The listing builds one solid part. Answer for the finished solid, in the listing's coordinates (mm). Face numbers are marked on the shaded views. Give positions to 0.01 mm unless a question says otherwise; leave off trailing zeros. Loops run counter-clockwise (first coordinate to the right, second up) from the corner with the lowest first, then second, coordinate; pieces in that order, holes last. Notation, with made-up numbers: M 39,-25.5 L 88,-25.5 A8 cw 88,-13.5 Z; hole C 34,37 d4. An arc over 180 degrees is marked long. Use one line per item in the form item = value. Start each with the question number.
1. The part is cut by section B-B (z = 1.75). Write down the section's boundary in (x, y), and give its area (3 significant figures).
2. The mould has two halves that part along X. Classify the marked faces 1, 2, 3 and 4: released by +X, released by -X, zero draft, split by the parting line, or undercut.
3. The part is cut by section C-C (y = 5). Write down the section's boundary in (x, z).
4. The part is cut by section A-A (y = 15). Write down the section's boundary in (x, z).
5. Each of these flat-tipped pins is pushed along its axis until it touches: pin 1 Ø2 at (x, y) = (1.5, 15.5) entering from -Z; pin 2 Ø12 at (x, y) = (4, 26.5) entering from -Z; pin 3 Ø2.5 at (x, y) = (5, -5) entering from +Z; pin 4 Ø1.8 at (x, y) = (-5, -5) entering from -Z. Where does it stop, or does it pass through?
6. Straight lines are drawn through the part: line 1 (Y direction, x = 0, z = 3.85); line 2 (Y direction, x = 0, z = 1.7); line 3 (X direction, y = 5, z = 2.2). For each, find the intervals that lie inside material, in ascending order. Write a range as from..to.
7. The part is cut by section D-D (x = -0.5). Write down the section's boundary in (y, z).
from build123d import *

# Parameters (mm, degrees)
SKETCH2_R           = 10
SKETCH2_R_2         = 1
SKETCH2_R_3         = 1.5
BOSS_EXTRUDE1_DEPTH = 5
SKETCH5_R           = 2
SKETCH5_R_2         = 1
CUT_EXTRUDE2_DEPTH  = 2
SKETCH6_R           = 3.5
CUT_EXTRUDE3_DEPTH  = 3


with BuildPart() as part:
    # Sketch2 → Boss-Extrude1 (new body)
    # profile 1 of 2: a face of its own
    with BuildSketch(Plane.XY):
        Circle(SKETCH2_R)
        with Locations((5, -5)):
            Circle(SKETCH2_R_2, mode=Mode.SUBTRACT)
        with Locations((-5, -5)):
            Circle(SKETCH2_R_2, mode=Mode.SUBTRACT)
        with Locations((5, 5)):
            Circle(SKETCH2_R_2, mode=Mode.SUBTRACT)
        with Locations((-5, 5)):
            Circle(SKETCH2_R_2, mode=Mode.SUBTRACT)
    # profile 2 of 2: a face of its own
    with BuildSketch(Plane.XY):
        with BuildLine():
            Line((-10, 40), (-10, 0))
            ThreePointArc((-10, 0), (0, 10), (10, 0))
            Line((10, 0), (10, 40))
            Line((10, 40), (-10, 40))
        make_face()
        with Locations((0, 15)):
            Circle(SKETCH2_R_3, mode=Mode.SUBTRACT)
        with Locations((0, 35)):
            Circle(SKETCH2_R_3, mode=Mode.SUBTRACT)
    extrude(amount=BOSS_EXTRUDE1_DEPTH)

    # Sketch5 → Cut-Extrude2 (cut)
    with BuildSketch(Plane.XY.offset(5)):
        with Locations((-5, 5)):
            Circle(SKETCH5_R)
        with Locations((5, 5)):
            Circle(SKETCH5_R)
        with Locations((5, -5)):
            Circle(SKETCH5_R)
        with Locations((-5, -5)):
            Circle(SKETCH5_R)
        with Locations((0, 3)):
            Circle(SKETCH5_R_2)
        with Locations((-3, 0)):
            Circle(SKETCH5_R_2)
        with Locations((3, 0)):
            Circle(SKETCH5_R_2)
        with Locations((0, -3)):
            Circle(SKETCH5_R_2)
    extrude(amount=-CUT_EXTRUDE2_DEPTH, mode=Mode.SUBTRACT)

    # Sketch6 → Cut-Extrude3 (cut)
    with BuildSketch(Plane(origin=(0, 0, 0), x_dir=(-1, 0, 0), z_dir=(0, 0, -1))):
        with Locations((0, 35)):
            Circle(SKETCH6_R)
        with Locations((0, 15)):
            Circle(SKETCH6_R)
    extrude(amount=-CUT_EXTRUDE3_DEPTH, mode=Mode.SUBTRACT)


solid = part.part
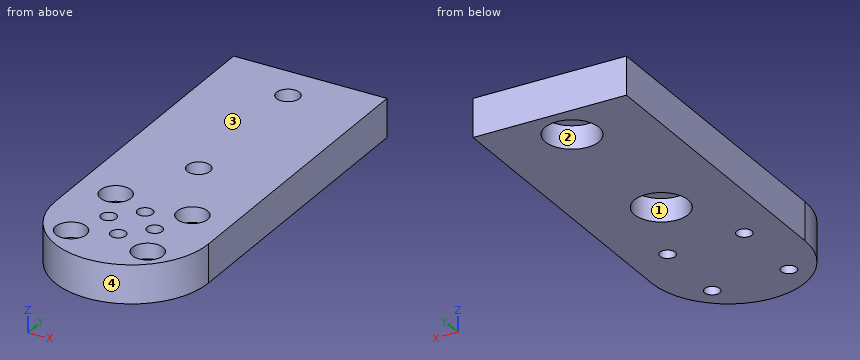
Derived:
q1.outline = M -10,0 A10 ccw 10,0 L 10,40 L -10,40 Z; hole C -5,-5 d2; hole C -5,5 d2; hole C 0,15 d7; hole C 0,35 d7; hole C 5,-5 d2; hole C 5,5 d2
q1.area = 868 mm2
q2.face_1 = undercut
q2.face_2 = undercut
q2.face_3 = zero draft
q2.face_4 = split by the parting line
q3.outline = M -10,0 L -6,0 L -6,3 L -7,3 L -7,5 L -10,5 Z; M -4,0 L 4,0 L 4,3 L 3,3 L 3,5 L -3,5 L -3,3 L -4,3 Z; M 6,0 L 10,0 L 10,5 L 7,5 L 7,3 L 6,3 Z
q4.outline = M -10,0 L -3.5,0 L -3.5,3 L -1.5,3 L -1.5,5 L -10,5 Z; M 1.5,3 L 3.5,3 L 3.5,0 L 10,0 L 10,5 L 1.5,5 Z
q5.pin_1 = 3
q5.pin_2 = 0
q5.pin_3 = 3
q5.pin_4 = through
q6.line_1 = -10..-4, -2..2, 4..13.5, 16.5..33.5, 36.5..40
q6.line_2 = -10..11.5, 18.5..31.5, 38.5..40
q6.line_3 = -10..-6, -4..4, 6..10
q7.outline = M -9.99,0 L 11.54,0 L 11.54,3 L 13.59,3 L 13.59,5 L 3.87,5 L 3.87,3 L 2.13,3 L 2.13,5 L -2.13,5 L -2.13,3 L -3.87,3 L -3.87,5 L -9.99,5 Z; M 16.41,3 L 18.46,3 L 18.46,0 L 31.54,0 L 31.54,3 L 33.59,3 L 33.59,5 L 16.41,5 Z; M 36.41,3 L 38.46,3 L 38.46,0 L 40,0 L 40,5 L 36.41,5 Z
